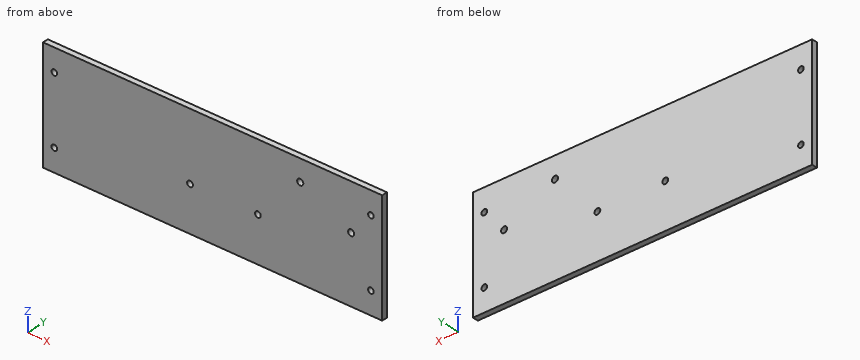
Autodesk Inventor part; units mm, degrees
ref_plane "YZ Plane" through (0, 0, 0) normal (1, 0, 0) x (0, 1, 0)
ref_plane "XZ Plane" through (0, 0, 0) normal (0, 1, 0) x (-1, 0, 0)
ref_plane "XY Plane" through (0, 0, 0) normal (0, 0, 1) x (1, 0, 0)
sketch "Sketch1" plane through (0, 0, 0) normal (0, 1, 0) x (-1, 0, 0)
  line L0 (0, 0) -> (381, 0)
  line L1 (381, 0) -> (381, -127)
  line L2 (381, -127) -> (0, -127)
  line L3 (0, -127) -> (0, 0)
  dimension "d0" = 381
  dimension "d1" = 127
extrude "Extrusion1" add sketch "Sketch1" along normal blind 6.35
sketch "Sketch2" plane through (0, 6.35, 0) normal (0, 1, 0) x (1, 0, 0)
  line L0 (0, 0) -> (0, 127)
  line L1 (0, 127) -> (-381, 127)
  line L2 (-381, 127) -> (-381, 0)
  point P0 (-368.3, 101.6)
  point P1 (-368.3, 25.4)
  point P2 (-12.7, 101.6)
  point P3 (-12.7, 25.4)
  dimension "d4" = 12.7
  dimension "d5" = 12.7
  dimension "d6" = 76.2
  dimension "d7" = 25.4
hole "Hole1" at (-368.3, 6.35, -101.6) at (-368.3, 6.35, -25.4) at (-12.7, 6.35, -101.6) at (-12.7, 6.35, -25.4) direction (0, -1, 0) diameter 6.35 end through all
sketch "Sketch3" plane through (0, 6.35, 0) normal (0, 1, 0) x (1, 0, 0)
  line L0 (0, 127) -> (-381, 127)
  line L1 (-381, 127) -> (-381, 0)
  point P0 (-215.9, 76.2)
  point P1 (-139.7, 76.2)
  dimension "d15" = 76.2
  dimension "d16" = 50.8
  dimension "d17" = 165.1
hole "Hole2" at (-215.9, 6.35, -76.2) at (-139.7, 6.35, -76.2) direction (0, -1, 0) diameter 6.5278 end through all
sketch "Sketch4" plane through (0, 6.35, 0) normal (0, 1, 0) x (1, 0, 0)
  line L0 (-381, 0) -> (0, 0)
  line L1 (0, 0) -> (0, 127)
  point P0 (-92.075, 24.13)
  point P1 (-34.925, 52.07)
  dimension "d25" = 57.15
  dimension "d26" = 27.94
  dimension "d27" = 24.13
  dimension "d28" = 34.925
hole "Hole3" at (-92.075, 6.35, -24.13) at (-34.925, 6.35, -52.07) direction (0, -1, 0) diameter 6.858 end through all
properties part number "Power Mount Plate" material "Aluminum 6061"
For this review, take the finished solid that the model builds, in its own axes (mm). Round coordinates to 2 decimals unless told otherwise and drop trailing zeros. Write each loop counter-clockwise with the first axis right and the second up, starting at its lowest first coordinate (ties: lowest second). Pieces come first, ordered by that corner, then holes. Notation, with made-up numbers: (69.25, -36) - (118.25, -36) arc R17 ccw to (118.25, -8) - close; hole circle Ø11 at (-24, 88.25). An arc over 180 degrees is marked (long way). Put each result on its own line as item: value.
Q1. We need section C-C (z = -76.2). Give the boundary of the cut face in (x, y), and give its area (3 significant figures).
Solved:
outline: (-381, 0) - (-219.16, 0) - (-219.16, 6.35) - (-381, 6.35) - close; (-212.64, 0) - (-142.96, 0) - (-142.96, 6.35) - (-212.64, 6.35) - close; (-136.44, 0) - (0, 0) - (0, 6.35) - (-136.44, 6.35) - close
area: 2,340 mm2
Q2. We need section B-B (x = -215.9). Give the boundary of the cut face in (y, z), and give its area (3 significant figures).
Solved:
outline: (0, -127) - (6.35, -127) - (6.35, -79.46) - (0, -79.46) - close; (0, -72.94) - (6.35, -72.94) - (6.35, 0) - (0, 0) - close
area: 765 mm2
Q3. Wall thickness on probe 1 along X at (y, z) = (4, -76.2); probe 2 along X at (y, z) = (5.25, -101.6) (3 decimals); probe 3 along Z at (x, y) = (-12.7, 2.75) (3 decimals): over which ranges is each line inside the solid? List them lowest first.
Solved:
probe 1: x = -381 to -219.16, -212.64 to -142.96, -136.44 to 0
probe 2: x = -381 to -371.475, -365.125 to -15.875, -9.525 to 0
probe 3: z = -127 to -104.775, -98.425 to -28.575, -22.225 to 0
Q4. We need section A-A (z = -52.07). Give the boundary of the cut face in (x, y), and give its area (3 significant figures).
Solved:
outline: (-381, 0) - (-38.35, 0) - (-38.35, 6.35) - (-381, 6.35) - close; (-31.5, 0) - (0, 0) - (0, 6.35) - (-31.5, 6.35) - close
area: 2,380 mm2
